```python
from build123d import *
from build123d.topology import SkipClean

# Parameters (mm, degrees)
SKETCH1_R             = 2.5
SKETCH1_R_2           = 1.4
BOSS_EXTRUDE1_DEPTH   = 6.3
BOSS_EXTRUDE1_2_DEPTH = 6.3
BOSS_EXTRUDE1_3_DEPTH = 6.3
BOSS_EXTRUDE1_4_DEPTH = 6.3
SKETCH2_R             = 1.4
SKETCH2_R_2           = 7
BOSS_EXTRUDE2_DEPTH   = 1


with BuildPart() as part:
    # Sketch1 → Boss-Extrude1 (new body)
    with BuildSketch(Plane.XY):
        with Locations((-7.071067812, 7.071067812)):
            Circle(SKETCH1_R)
        with Locations((-7.071067812, 7.071067812)):
            Circle(SKETCH1_R_2, mode=Mode.SUBTRACT)
    extrude(amount=BOSS_EXTRUDE1_DEPTH)



with BuildPart() as body_2:
    # Sketch1 → Boss-Extrude1 2 (new body)
    with BuildSketch(Plane.XY):
        with Locations((7.071067812, 7.071067812)):
            Circle(SKETCH1_R)
        with Locations((7.071067812, 7.071067812)):
            Circle(SKETCH1_R_2, mode=Mode.SUBTRACT)
    extrude(amount=BOSS_EXTRUDE1_2_DEPTH)


with BuildPart() as body_3:
    # Sketch1 → Boss-Extrude1 3 (new body)
    with BuildSketch(Plane.XY):
        with Locations((7.071067812, -7.071067812)):
            Circle(SKETCH1_R)
        with Locations((7.071067812, -7.071067812)):
            Circle(SKETCH1_R_2, mode=Mode.SUBTRACT)
    extrude(amount=BOSS_EXTRUDE1_3_DEPTH)


with BuildPart() as body_4:
    # Sketch1 → Boss-Extrude1 4 (new body)
    with BuildSketch(Plane.XY):
        with Locations((-7.071067812, -7.071067812)):
            Circle(SKETCH1_R)
        with Locations((-7.071067812, -7.071067812)):
            Circle(SKETCH1_R_2, mode=Mode.SUBTRACT)
    extrude(amount=BOSS_EXTRUDE1_4_DEPTH)


with BuildPart() as part_1:
    with SkipClean():  # the faces are left unmerged after this step: merging them gives an invalid solid
        add(part.part)

        add(body_2.part)  # Boss-Extrude2 merges body 2

        add(body_3.part)  # Boss-Extrude2 merges body 3

        add(body_4.part)  # Boss-Extrude2 merges body 4
        # Sketch2 → Boss-Extrude2 (add)
        with BuildSketch(Plane.XY.offset(6.3)):
            with BuildLine():
                Line((-9.571067812, 7.071067812), (-9.571067812, -7.071067812))
                ThreePointArc((-9.571067812, -7.071067812), (-8.838834765, -8.838834765), (-7.071067812, -9.571067812))
                Line((-7.071067812, -9.571067812), (7.071067812, -9.571067812))
                ThreePointArc((7.071067812, -9.571067812), (8.838834765, -8.838834765), (9.571067812, -7.071067812))
                Line((9.571067812, -7.071067812), (9.571067812, 7.071067812))
                ThreePointArc((9.571067812, 7.071067812), (8.838834765, 8.838834765), (7.071067812, 9.571067812))
                Line((7.071067812, 9.571067812), (-7.071067812, 9.571067812))
                ThreePointArc((-7.071067812, 9.571067812), (-8.838834765, 8.838834765), (-9.571067812, 7.071067812))
            make_face()
            with Locations((7.071067812, -7.071067812)):
                Circle(SKETCH2_R, mode=Mode.SUBTRACT)
            with Locations((7.071067812, 7.071067812)):
                Circle(SKETCH2_R, mode=Mode.SUBTRACT)
            with Locations((-7.071067812, -7.071067812)):
                Circle(SKETCH2_R, mode=Mode.SUBTRACT)
            with Locations((-7.071067812, 7.071067812)):
                Circle(SKETCH2_R, mode=Mode.SUBTRACT)
            Circle(SKETCH2_R_2, mode=Mode.SUBTRACT)
        extrude(amount=BOSS_EXTRUDE2_DEPTH)


solid = part_1.part
```
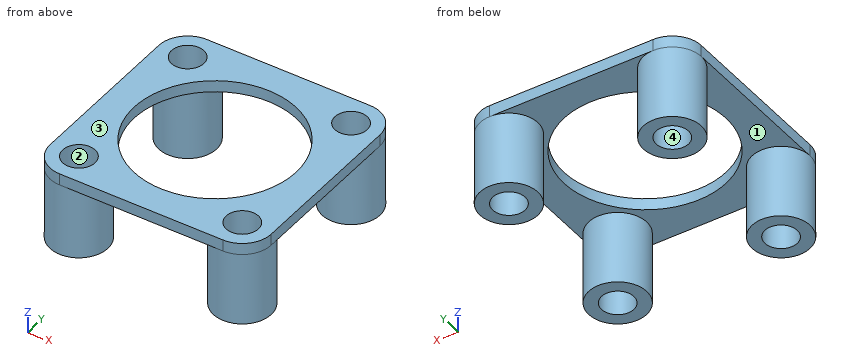
Here's how the part is built. I have some questions about the finished solid (model axes, mm). Face numbers are marked on the shaded views. A direction names the side the tool comes from. Give positions to 0.01 mm unless a question says otherwise; leave off trailing zeros. Write each loop counter-clockwise with the first axis right and the second up, starting at its lowest first coordinate (ties: lowest second). Pieces come first, ordered by that corner, then holes.
(1) If I drill on L1, parallel to X at y = 7, z = 3.75; L2, parallel to Y at x = 0, z = 7.1; L3, parallel to Y at x = -7.25, z = 5.5, over which ranges is the centre line in solid material (lowest first)?
Output values:
L1: x = -9.57 to -8.47, -5.67 to -4.57, 4.57 to 5.67, 8.47 to 9.57
L2: y = -9.57 to -7, 7 to 9.57
L3: y = -9.56 to -8.46, -5.68 to -4.58, 4.58 to 5.68, 8.46 to 9.56
(2) On a 3-axis mill with a long thin cutter (end or side, diameter ignored), from which of +Z, -Z, +X, -X, +Y, -Y can I reach the whole of each face in a straight line? I mean the marked faces 1 and 2. Say none if no direction works.
Output values:
face 1: -Z
face 2: +Z, -Z
(3) Thinking about a two-plate mould opening in Y: for the marked faces 3 and 4, which applies, pulls with the +Y half, pulls with the -Y half, needs draft (parallel to the pull), parting line crosses it, or undercut?
Output values:
face 3: needs draft
face 4: undercut
(4) Imagine slicing it at B-B, the plane y = 0. Write out the boundary of the cut face in (x, z).
Output values:
outline: (-9.57, 6.3) - (-7, 6.3) - (-7, 7.3) - (-9.57, 7.3) - close; (7, 6.3) - (9.57, 6.3) - (9.57, 7.3) - (7, 7.3) - close
(5) Will these pins go through, and if not, where does the flat tip stop? pin 1 (4 mm diameter, centred on x = 5, y = 1, fed in from +Z); pin 2 (1 mm diameter, centred on x = -4.5, z = 4.5, fed in from -Y); pin 3 (6 mm diameter, centred on x = 1, y = -7, fed in from -Z).
Output values:
pin 1: stops at z = 7.3
pin 2: stops at y = -8.47
pin 3: stops at z = 6.3
(6) Imagine slicing it at D-D, the plane x = -7.5. Write out the boundary of the cut face in (y, z), and give its area (3 significant figures).
Output values:
outline: (-9.53, 0) - (-8.4, 0) - (-8.4, 7.3) - (-9.53, 7.3) - close; (-5.74, 0) - (-4.61, 0) - (-4.61, 6.3) - (4.61, 6.3) - (4.61, 0) - (5.74, 0) - (5.74, 7.3) - (-5.74, 7.3) - close; (8.4, 0) - (9.53, 0) - (9.53, 7.3) - (8.4, 7.3) - close
area: 42.2 mm2
(7) Imagine slicing it at A-A, the plane z = 5.5. Write out the boundary of the cut face in (x, y).
Output values:
outline: circle Ø5 at (-7.07, -7.07); circle Ø5 at (-7.07, 7.07); circle Ø5 at (7.07, -7.07); circle Ø5 at (7.07, 7.07); hole circle Ø2.8 at (-7.07, -7.07); hole circle Ø2.8 at (-7.07, 7.07); hole circle Ø2.8 at (7.07, -7.07); hole circle Ø2.8 at (7.07, 7.07)
